Geometry check sheet. Reference: the model listing, model coordinates, mm. Face numbers are marked on the shaded views. A direction names the side the tool comes from. Coordinates: 2 decimals unless noted, no trailing zeros. Order: outer loops, then holes, each group sorted by start corner. A loop starts at its lowest first (then second) coordinate and runs counter-clockwise, first axis right, second up. Notation, with made-up numbers: (61, 14.25) - (117, 14.25) arc R12 ccw to (117, 21.25) - close; hole circle Ø3 at (87, 34). An arc over 180 degrees is marked (long way). Return JSON: item names as keys, results as strings. Group by question number.
Item 1: Section check B-B on z = 5. Enter the section's corners in (x, y).
Item 2: Section check A-A on x = 0. Enter the section's corners in (y, z), then the cut area to 3 significant figures.
Item 3: Scan lines: probe 1 along X at (y, z) = (0, 0.45); probe 2 along Z at (x, y) = (10.4, 0); probe 3 along X at (y, z) = (5.5, 14.75). Record each from-to range of solid material in increasing order.
Item 4: Gauge pin test, flat ends, axial feed: pin 1 (5 mm diameter, centred on y = 0, z = 9.6, fed in from +X); pin 2 (2 mm diameter, centred on x = -16, y = 4, fed in from +Z); pin 3 (2.5 mm diameter, centred on x = -12, z = 5.5, fed in from +Y). Record the tip position at first contact, or that the pin passes through.
Item 5: Draft check along X on the marked faces 4, 5 and 6. Enter one of: pulls with the +X half, pulls with the -X half, needs draft (parallel to the pull), parting line crosses it, or undercut.
Item 6: Section check D-D on y = 0. Give the number of separate pieces and of enclosed holes in the cut face, then the cut area to 3 significant figures.
Item 7: Tool access check on the marked faces 1, 2 and 3. Record the directions out of +Z, -Z, +X, -X, +Y, -Y that give a thin tool (end or side, any length) a straight path to the whole face; none if there is none.
Item 8: Section check C-C on y = 10. Enter the section's corners in (x, z), then the cut area to 3 significant figures.
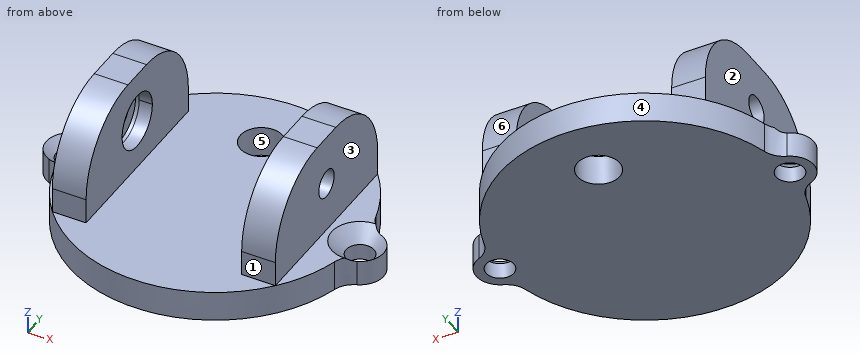
from build123d import *

# Parameters (mm, degrees)
F1_DEPTH             = 3.6
F2_R                 = 2.8
F4_D                 = 3.3
F4_DEPTH             = 20
F4_CSINK_D           = 6.72
F4_CSINK_ANGLE       = 90
F4_TIP               = 0.9914200214
F3_R                 = 2.5
F5_DEPTH             = 3.6
F3_W                 = 4
F3_H                 = 22
F6_DEPTH             = 12
F9_D                 = 3.3
F9_DEPTH             = 20
F9_CBORE_D           = 6.5
F9_CBORE_DEPTH       = 2
F9_TIP               = 0.9914200214
F9_ON_F7_D           = 3.3
F9_ON_F7_DEPTH       = 20
F9_ON_F7_CBORE_D     = 6.5
F9_ON_F7_CBORE_DEPTH = 2
F9_ON_F7_TIP         = 0.9914200214
F10_R                = 9


with BuildPart() as f1:
    # F0 (on Top) → F1 (new body)
    with BuildSketch(Plane.XY):
        with BuildLine():
            ThreePointArc((16.9720930233, -2.7907093023), (20, 0), (16.9720930233, 2.7907093023))
            ThreePointArc((16.9720930233, 2.7907093023), (0, 17.2), (-16.9720930233, 2.7907093023))
            ThreePointArc((-16.9720930233, 2.7907093023), (-20, 0), (-16.9720930233, -2.7907093023))
            ThreePointArc((-16.9720930233, -2.7907093023), (0, -17.2), (16.9720930233, -2.7907093023))
        make_face()
    extrude(amount=F1_DEPTH)

    # F2
    f2_edges = [f1.edges().sort_by_distance(p)[0] for p in [
        (-16.972093, -2.790709, 1.8),
        (16.972093, -2.790709, 1.8),
        (16.972093, 2.790709, 1.8),
        (-16.972093, 2.790709, 1.8),
    ]]
    fillet(f2_edges, radius=F2_R)

    # F4
    with Locations(Plane.XY.offset(3.6)):
        with Locations((-17.2, 0), (17.2, 0)):
            CounterSinkHole(F4_D / 2, F4_CSINK_D / 2, depth=F4_DEPTH, counter_sink_angle=F4_CSINK_ANGLE)
            with Locations((0, 0, -(F4_DEPTH + F4_TIP / 2))):  # 118° drill point
                Cone(0, F4_D / 2, F4_TIP, mode=Mode.SUBTRACT)

    # F3 (on face) → F5 (cut, through all)
    with BuildSketch(Plane.XY.offset(3.6)):
        with Locations((0, 10)):
            Circle(F3_R)
    extrude(amount=-F5_DEPTH, mode=Mode.SUBTRACT)

    # F3 (on face) → F6 (join)
    with BuildSketch(Plane.XY.offset(3.6)):
        with Locations((-11.2227077409, 0)):
            Rectangle(F3_W, F3_H)
        with Locations((11.2227077409, 0)):
            Rectangle(F3_W, F3_H)
    extrude(amount=F6_DEPTH)

    # F9
    with Locations(Plane(origin=(9.2227077409, 0, 0), x_dir=(0, -1, 0), z_dir=(-1, 0, 0))):
        with Locations((0, 9.6)):
            CounterBoreHole(F9_D / 2, F9_CBORE_D / 2, F9_CBORE_DEPTH, depth=F9_DEPTH)
            with Locations((0, 0, -(F9_DEPTH + F9_TIP / 2))):  # 118° drill point
                Cone(0, F9_D / 2, F9_TIP, mode=Mode.SUBTRACT)

    # F9 on F7
    with Locations(Plane.YZ.offset(-9.2227077409)):
        with Locations((0, 9.6)):
            CounterBoreHole(F9_ON_F7_D / 2, F9_ON_F7_CBORE_D / 2, F9_ON_F7_CBORE_DEPTH, depth=F9_ON_F7_DEPTH)
            with Locations((0, 0, -(F9_ON_F7_DEPTH + F9_ON_F7_TIP / 2))):  # 118° drill point
                Cone(0, F9_ON_F7_D / 2, F9_ON_F7_TIP, mode=Mode.SUBTRACT)

    # F10
    f10_edges = [f1.edges().sort_by_distance(p)[0] for p in [
        (11.222708, 11, 15.6),
        (-11.222708, 11, 15.6),
        (-11.222708, -11, 15.6),
        (11.222708, -11, 15.6),
    ]]
    fillet(f10_edges, radius=F10_R)


solid = f1.part
Computed:
{
 "1": {"outline": "(-13.22, -11) - (-9.22, -11) - (-9.22, 11) - (-13.22, 11) - close; (9.22, -11) - (13.22, -11) - (13.22, 11) - (9.22, 11) - close"},
 "2": {"outline": "(-17.2, 0) - (7.5, 0) - (7.5, 3.6) - (-17.2, 3.6) - close; (12.5, 0) - (17.2, 0) - (17.2, 3.6) - (12.5, 3.6) - close", "area": "106 mm²"},
 "3": {"probe 1": "x = -20 to -18.85, -15.55 to 15.55, 18.85 to 20", "probe 2": "z = 0 to 6.35, 12.85 to 15.6", "probe 3": "x = -13.22 to -9.22, 9.22 to 13.22"},
 "4": {"pin 1": "stops at x = 13.22", "pin 2": "stops at z = 3.6", "pin 3": "stops at y = 11"},
 "5": {"face 4": "parting line crosses it", "face 5": "undercut", "face 6": "needs draft"},
 "6": {"separate pieces": "5", "enclosed holes": "0", "area": "172 mm²"},
 "7": {"face 1": "+Z, +X, -X, -Y", "face 2": "+Z, -X, +Y, -Y", "face 3": "+Z, +X, +Y, -Y"},
 "8": {"outline": "(-13.99, 0) - (-2.5, 0) - (-2.5, 3.6) - (-9.22, 3.6) - (-9.22, 10.72) - (-13.22, 10.72) - (-13.22, 3.6) - (-13.99, 3.6) - close; (2.5, 0) - (13.99, 0) - (13.99, 3.6) - (13.22, 3.6) - (13.22, 10.72) - (9.22, 10.72) - (9.22, 3.6) - (2.5, 3.6) - close", "area": "140 mm²"}
}
